from build123d import *

# Parameters (mm, degrees)
F0_W     = 50.8
F0_H     = 50.8
F0_R     = 3.146652
F0_R_2   = 19.05
F1_DEPTH = 25.4
F2_DEPTH = 12.7


with BuildPart() as f1:
    # F0 (on Front) → F1 (new body)
    with BuildSketch(Plane.XZ):
        with Locations((25.4, 25.4)):
            Rectangle(F0_W, F0_H)
        with Locations((9.101667, 8.043333)):
            Circle(F0_R, mode=Mode.SUBTRACT)
        with Locations((20.43549, 29.136131)):
            Circle(F0_R_2, mode=Mode.SUBTRACT)
    extrude(amount=F1_DEPTH)

    # F0 (on Front) → F2 (join)
    with BuildSketch(Plane.XZ):
        with Locations((9.101667, 8.043333)):
            Circle(F0_R)
    extrude(amount=F2_DEPTH)


solid = f1.part
The listing builds one solid part. Answer for the finished solid, in the listing's coordinates (mm). A direction names the side the tool comes from. Coordinates: 2 decimals unless noted, no trailing zeros. Write each loop counter-clockwise with the first axis right and the second up, starting at its lowest first coordinate (ties: lowest second). Pieces come first, ordered by that corner, then holes. Notation, with made-up numbers: M 34,-39 L 54,-39 A20 ccw 54,-3 Z; hole C 52.5,31.5 d1. An arc over 180 degrees is marked long. Put each result on its own line as item: value. Start each with the question number.
1. A flat-ended cylindrical pin translates along its axis: P1, Ø1.9, axis at x = 9.5, z = 9, coming from the -Y side. Find the tip coordinate at first contact, or state that the pin passes through.
2. Consider line 1 (Z direction, x = 8, y = -17); line 2 (Z direction, x = 27, y = -17.75); line 3 (X direction, y = -11.75, z = 17.5). Determine where each line is inside the solid, lowest interval first. Write a range as from..to.
3. A cutting plane is placed at B-B on z = 25.5. Write down the section's boundary in (x, y), then the cut area to 3 significant figures.
4. A cutting plane is placed at A-A on x = 32.5. Write down the section's boundary in (y, z).
5. Which of the six approach directions +Z, -Z, +X, -X, +Y, -Y give full straight-line access (tool end or side, diameter ignored) to faces 5 (the flat face through (50.8, -13, 25)), 6 (the cylindrical face through (5.958, -18.961, 8.182))?
6. A cutting plane is placed at C-C on y = -4.25. Write down the section's boundary in (x, z).
7. For a pull along Z with two mould halves and no side action, classify faces 1 (the flat face through (25, -13, 0)), 2 (the flat face through (0, -13, 25)), 3 (the flat face through (25, -13, 50.8)), 4 (the flat face through (9, -12.7, 8)) as pulls with the +Z half, pulls with the -Z half, needs draft (parallel to the pull), parting line crosses it, or undercut.
8. A cutting plane is placed at D-D on y = -15.75. Write down the section's boundary in (x, z).
Resolved:
1. P1: stops at y = -12.7
2. line 1: z = 0..5.1, 10.99..14.7, 43.57..50.8
2. line 2: z = 0..11.25, 47.02..50.8
2. line 3: x = 0..5.35, 35.52..50.8
3. outline: M 0,-25.4 L 1.74,-25.4 L 1.74,0 L 0,0 Z; M 39.14,-25.4 L 50.8,-25.4 L 50.8,0 L 39.14,0 Z
3. area: 340 mm2
4. outline: M -25.4,0 L 0,0 L 0,14.39 L -25.4,14.39 Z; M -25.4,43.88 L 0,43.88 L 0,50.8 L -25.4,50.8 Z
5. face 5: +Z, -Z, +X, +Y, -Y
5. face 6: -Y
6. outline: M 0,0 L 50.8,0 L 50.8,50.8 L 0,50.8 Z; hole C 20.44,29.14 d38.1
7. face 1: pulls with the -Z half
7. face 2: needs draft
7. face 3: pulls with the +Z half
7. face 4: undercut
8. outline: M 0,0 L 50.8,0 L 50.8,50.8 L 0,50.8 Z; hole C 20.44,29.14 d38.1; hole C 9.1,8.04 d6.29
